Job drawing, mm, ordinate dimensions from the low corner. One solid piece. A direction names the side the tool comes from. Give positions to 0.01 mm unless a question says otherwise; leave off trailing zeros. Order: outer loops, then holes, each group sorted by start corner. A loop starts at its lowest first (then second) coordinate and runs counter-clockwise, first axis right, second up. Notation, with made-up numbers: (18.5, 32.5) -> (48.5, 32.5) arc R27 cw to (48.5, 51.5) -> close; hole circle Ø3 at (79, -5). An arc over 180 degrees is marked (long way). Write item = value, one per line. Start each with the question number.
(1) Which spindle directions (+Z, -Z, +X, -X, +Y, -Y) get a long thin tool onto all of the face, cutting with end or side? Do the marked faces 4 and 5. Say none if no direction does.
(2) Two-plate mould, pull along Y, no slides. Class the marked faces 1, 2 and 3: pulls with the +Y half, pulls with the -Y half, needs draft (parallel to the pull), parting line crosses it, or undercut.
(3) Saw through at D-D, the plane z = 3.05. List the corners of the cut face in (x, y).
(4) Probe line 1 along Y through (x, z) = (3, 0.65); line 2 along Z through (x, y) = (3.9, 4.9); line 3 along Z through (x, y) = (4.3, 3.15). List the from-to ranges inside material, lowest first. Write a range as from..to.
(5) Saw through at A-A, the plane x = 3. List the corners of the cut face in (y, z), then the cut area to 3 significant figures.
(6) Flat gauge pins, fed straight in: pin 1 (1.5 mm diameter, centred on x = 3.5, y = 1, fed in from +Z); pin 2 (1.5 mm diameter, centred on x = 4.5, z = 0.5, fed in from -Y); pin 3 (3.5 mm diameter, centred on x = 3, y = 3, fed in from -Z). Where does each tip first touch, or does it go through?
(7) Saw through at B-B, the plane z = 0.35. List the corners of the cut face in (x, y).
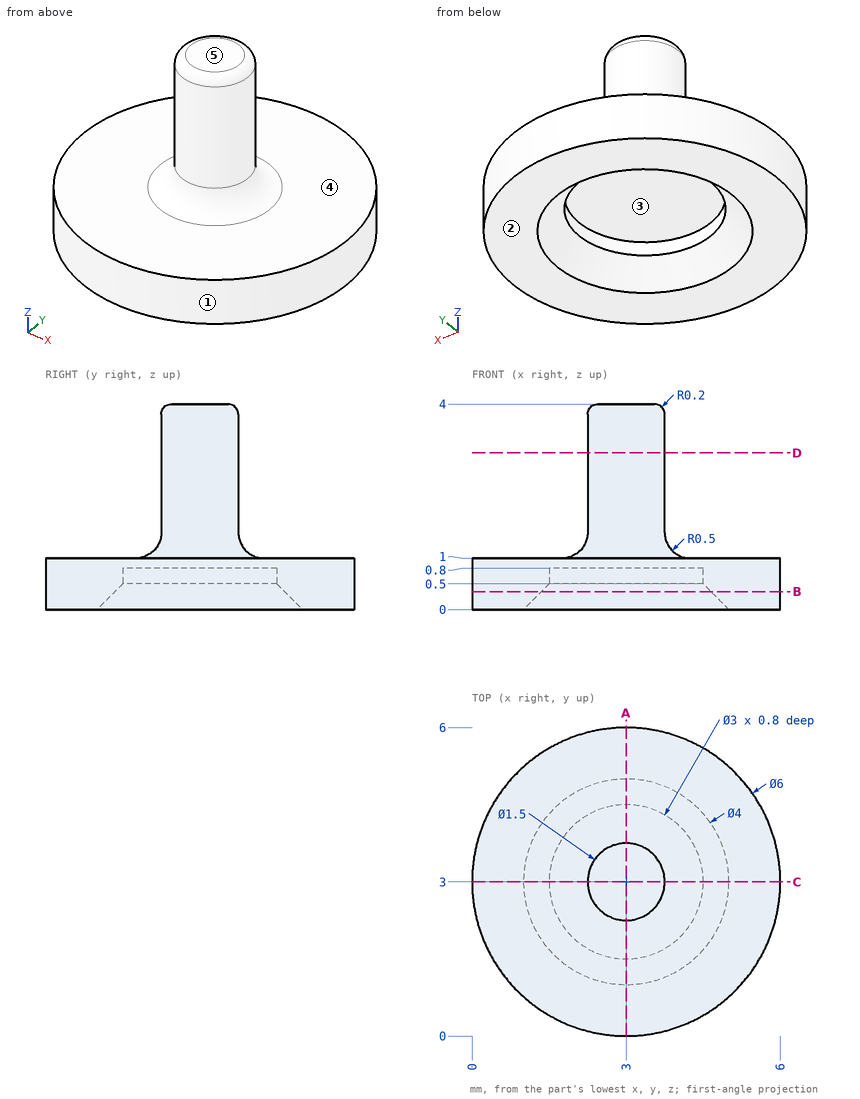
Results list:
q1.face_4 = +Z
q1.face_5 = +Z, +X, -X, +Y, -Y
q2.face_1 = parting line crosses it
q2.face_2 = needs draft
q2.face_3 = undercut
q3.outline = circle Ø1.5 at (3, 3)
q4.line_1 = 0..1.5, 4.5..6
q4.line_2 = 0..1
q4.line_3 = 0.8..1
q5.outline = (0, 0) -> (1, 0) -> (1.5, 0.5) -> (1.5, 0.8) -> (4.5, 0.8) -> (4.5, 0.5) -> (5, 0) -> (6, 0) -> (6, 1) -> (4.25, 1) arc R0.5 cw to (3.75, 1.5) -> (3.75, 3.8) arc R0.2 ccw to (3.55, 4) -> (2.45, 4) arc R0.2 ccw to (2.25, 3.8) -> (2.25, 1.5) arc R0.5 cw to (1.75, 1) -> (0, 1) -> close
q5.area = 7.94 mm^2
q6.pin_1 = 1
q6.pin_2 = 0.1
q6.pin_3 = 0.25
q7.outline = circle Ø6 at (3, 3); hole circle Ø3.3 at (3, 3)
